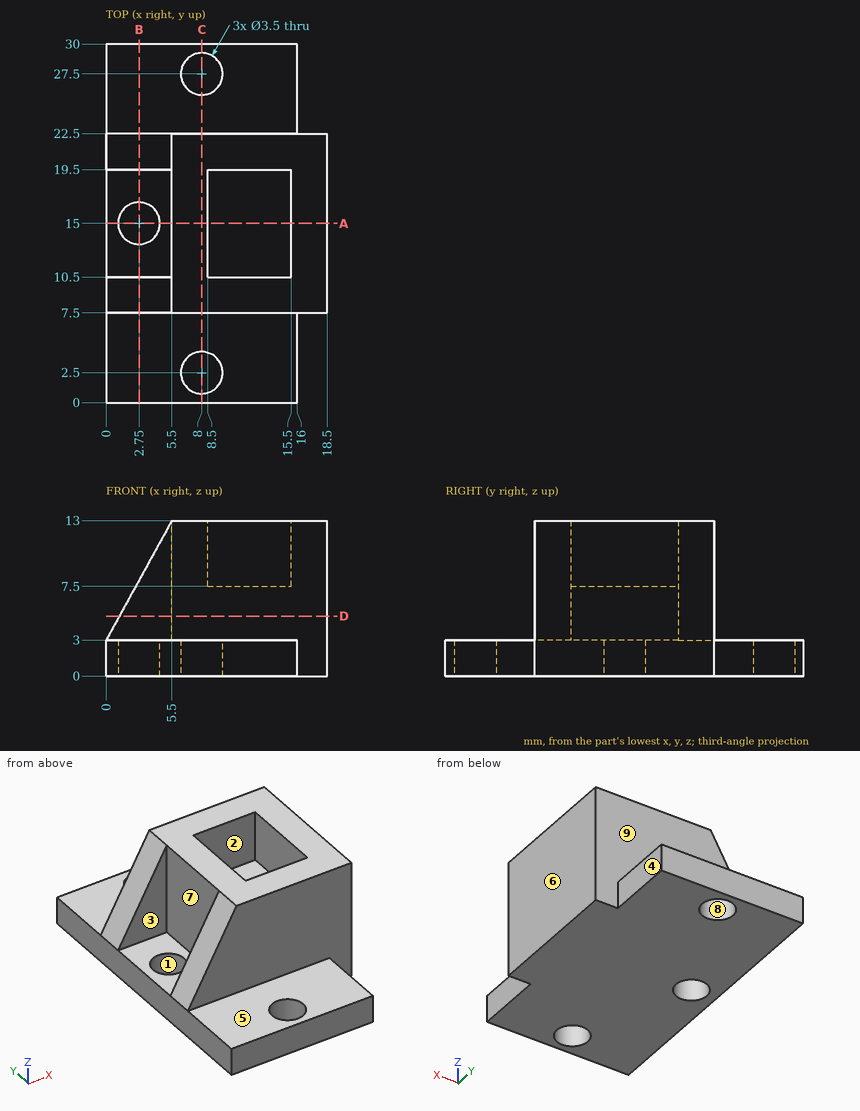
Could you check a few things on this drawing? It's one solid part, dimensions in mm from its lowest x, y, z. A direction names the side the tool comes from. Coordinates: 2 decimals unless noted, no trailing zeros. Order: outer loops, then holes, each group sorted by start corner. A loop starts at its lowest first (then second) coordinate and runs counter-clockwise, first axis right, second up. Notation, with made-up numbers: (-38, -31) - (6, -31) arc R29 ccw to (6, 8) - close; hole circle Ø7 at (-25.5, -31). An arc over 180 degrees is marked (long way). One line per question, with ' | ' between items.
(1) Suppose I cut it at D-D on z = 5. List the corners of the cut face in (x, y) for me.
Report:
outline: (1.1, 7.5) - (18.5, 7.5) - (18.5, 22.5) - (1.1, 22.5) - (1.1, 19.5) - (5.5, 19.5) - (5.5, 10.5) - (1.1, 10.5) - close
(2) For the marked faces 1, 2, 3, 4 and 5, which set-ups out of +Z, -Z, +X, -X, +Y, -Y let a thin tool reach every point of the face, with its end or its side?
Report:
face 1: +Z, -Z | face 2: +Z | face 3: +Z, -X | face 4: +Z, -Z, +X, +Y | face 5: +Z, +X, -X, -Y
(3) If I drill on L1, parallel to Y at x = 8, z = 1.1; L2, parallel to Y at x = 11.25, z = 8; L3, parallel to Y at x = 2.75, z = 1, over which ranges is the centre line in solid material (lowest first)?
Report:
L1: y = 0 to 0.75, 4.25 to 25.75, 29.25 to 30 | L2: y = 7.5 to 10.5, 19.5 to 22.5 | L3: y = 0 to 13.25, 16.75 to 30
(4) Suppose I cut it at B-B on x = 2.75. List the corners of the cut face in (y, z) for me, and give its area (4 significant figures).
Report:
outline: (0, 0) - (13.25, 0) - (13.25, 3) - (10.5, 3) - (10.5, 8) - (7.5, 8) - (7.5, 3) - (0, 3) - close; (16.75, 0) - (30, 0) - (30, 3) - (22.5, 3) - (22.5, 8) - (19.5, 8) - (19.5, 3) - (16.75, 3) - close | area: 109.5 mm2
(5) Suppose I cut it at C-C on x = 8. List the corners of the cut face in (y, z) for me, and give its area (3 significant figures).
Report:
outline: (0, 0) - (0.75, 0) - (0.75, 3) - (0, 3) - close; (4.25, 0) - (25.75, 0) - (25.75, 3) - (22.5, 3) - (22.5, 13) - (7.5, 13) - (7.5, 3) - (4.25, 3) - close; (29.25, 0) - (30, 0) - (30, 3) - (29.25, 3) - close | area: 219 mm2
(6) Suppose I cut it at A-A on y = 15. List the corners of the cut face in (x, z) for me, and give its area (4 significant figures).
Report:
outline: (0, 0) - (1, 0) - (1, 3) - (0, 3) - close; (4.5, 0) - (18.5, 0) - (18.5, 13) - (15.5, 13) - (15.5, 7.5) - (8.5, 7.5) - (8.5, 13) - (5.5, 13) - (5.5, 3) - (4.5, 3) - close | area: 136.5 mm2
(7) If we mould it in two halves opening along X, with no side actions, what happens to the marked faces 6, 7, 8 and 9? For each: pulls with the +X half, pulls with the -X half, needs draft (parallel to the pull), parting line crosses it, or undercut.
Report:
face 6: pulls with the +X half | face 7: pulls with the -X half | face 8: undercut | face 9: needs draft
(8) Will these pins go through, and if not, where does the flat tip stop? pin 1 (1.6 mm diameter, centred on y = 16, z = 10, fed in from -X); pin 2 (3 mm diameter, centred on x = 3.5, y = 16, fed in from +Z); pin 3 (1 mm diameter, centred on x = 13, y = 16.5, fed in from -Z); pin 4 (3.5 mm diameter, centred on y = 26, z = 1, fed in from +X).
Report:
pin 1: stops at x = 5.5 | pin 2: stops at z = 3 | pin 3: stops at z = 0 | pin 4: stops at x = 16
